from build123d import *

# Parameters (mm, degrees)
SZKIC1_R                    = 30
DODANIE_WYCI_GNI_CIE1_DEPTH = 200
SZKIC2_W                    = 50
SZKIC2_H                    = 60
DODANIE_WYCI_GNI_CIE2_DEPTH = 30
SZKIC3_W                    = 40
SZKIC3_H                    = 50
WYTNIJ_WYCI_GNI_CIE1_DEPTH  = 61


with BuildPart() as part:
    # Szkic1 → Dodanie-wyciągnięcie1 (new body)
    with BuildSketch(Plane.XY):
        Circle(SZKIC1_R)
    extrude(amount=DODANIE_WYCI_GNI_CIE1_DEPTH)

    # Szkic2 → Dodanie-wyciągnięcie2 (add, symmetric)
    with BuildSketch(Plane(origin=(0, 0, 0), x_dir=(0, 0, -1), z_dir=(1, 0, 0))):
        with Locations((-225, 0)):
            Rectangle(SZKIC2_W, SZKIC2_H)
    extrude(amount=DODANIE_WYCI_GNI_CIE2_DEPTH, both=True)

    # Szkic3 → Wytnij-wyciągnięcie1 (cut, through all)
    with BuildSketch(Plane(origin=(30, 0, 0), x_dir=(0, 0, -1), z_dir=(1, 0, 0))):
        with Locations((-226.037911192, -0.873923737)):
            Rectangle(SZKIC3_W, SZKIC3_H)
    extrude(amount=-WYTNIJ_WYCI_GNI_CIE1_DEPTH, mode=Mode.SUBTRACT)


solid = part.part
Read the model definition and answer for the solid it produces. Units are mm, in the model's axes. A direction names the side the tool comes from. Give positions to 0.01 mm unless a question says otherwise; leave off trailing zeros. Write each loop counter-clockwise with the first axis right and the second up, starting at its lowest first coordinate (ties: lowest second). Pieces come first, ordered by that corner, then holes. Notation, with made-up numbers: (36.5, 46.25) - (90.5, 46.25) arc R23 cw to (90.5, 68.25) - close; hole circle Ø6 at (75.5, 40.25). An arc over 180 degrees is marked (long way). Use CSV: the item, a comma, the result in double quotes. Start each with the question number.
Item 1: The part is cut by section C-C, the plane y = -16. Give the vertices of the cut face in (x, z), and give its area (3 significant figures).
Item 2: Consider line 1 (Z direction, x = 4, y = -9); line 2 (Y direction, x = 10.5, z = 207); line 3 (X direction, y = -1, z = 141.5). Determine where each line is inside the solid, lowest interval first.
Item 3: For faces 4 (the flat face through (0, -25.874, 226)), 5 (the flat face through (-23, -24, 200)), 6 (the flat face through (24, 23, 200)), 7 (the flat face through (23, -24, 200)), determine the directions among +Z, -Z, +X, -X, +Y, -Y from which every point of the face is accessible in a straight line to the end or side of a thin tool.
Item 4: Flat-ended cylindrical pins translate along their axes: P1, Ø5, axis at x = 2, z = 42.5, coming from the -Y side; P2, Ø10, axis at y = -21, z = 62.5, coming from the -X side; P3, Ø8, axis at y = -9, z = 66.5, coming from the -X side. Find the tip coordinate at first contact, or state that the pin passes through.
Item 5: The part is cut by section D-D, the plane z = 47.5. Give the vertices of the cut face in (x, y).
Item 6: The mould has two halves that part along Z. Classify faces 1 (the cylindrical face through (-29.97, 1.32, 98.6)), 2 (the flat face through (0, -1, 246.038)), 3 (the flat face through (0, 0, 0)): pulls with the +Z half, pulls with the -Z half, needs draft (parallel to the pull), parting line crosses it, or undercut.
Item 7: The part is cut by section A-A, the plane y = -3.5. Give the vertices of the cut face in (x, z).
Item 8: The part is cut by section B-B, the plane x = 10.5. Give the vertices of the cut face in (y, z).
Taken from the geometry:
1,outline,"(-30, 200) - (-25.38, 200) - (-25.38, 0) - (25.38, 0) - (25.38, 200) - (30, 200) - (30, 206.04) - (-30, 206.04) - close; (-30, 246.04) - (30, 246.04) - (30, 250) - (-30, 250) - close"
1,area,"10,800 mm2"
2,line 1,"0 to 206.04, 246.04 to 250"
2,line 2,"-30 to -25.87, 24.13 to 30"
2,line 3,"-29.98 to 29.98"
3,face 4,"+X, -X"
3,face 5,"-Z, -X, -Y"
3,face 6,"-Z, +X, +Y"
3,face 7,"-Z, +X, -Y"
4,P1,"y = -30"
4,P2,"x = -25.38"
4,P3,"x = -29.58"
5,outline,"circle Ø60 at (0, 0)"
6,face 1,"needs draft"
6,face 2,"undercut"
6,face 3,"pulls with the -Z half"
7,outline,"(-30, 200) - (-29.8, 200) - (-29.8, 0) - (29.8, 0) - (29.8, 200) - (30, 200) - (30, 206.04) - (-30, 206.04) - close; (-30, 246.04) - (30, 246.04) - (30, 250) - (-30, 250) - close"
8,outline,"(-30, 200) - (-28.1, 200) - (-28.1, 0) - (28.1, 0) - (28.1, 200) - (30, 200) - (30, 250) - (-30, 250) - close; hole (-25.87, 206.04) - (24.13, 206.04) - (24.13, 246.04) - (-25.87, 246.04) - close"
